Geometry check sheet. Reference: the model listing, model coordinates, mm. Face numbers are marked on the shaded views. A direction names the side the tool comes from. Coordinates: 2 decimals unless noted, no trailing zeros. Loops run counter-clockwise (first coordinate to the right, second up) from the corner with the lowest first, then second, coordinate; pieces in that order, holes last. Notation, with made-up numbers: (-4.5, -1.75) -> (38.5, -1.75) arc R36 cw to (38.5, 35.25) -> close; hole circle Ø3 at (85.5, 68.25). An arc over 180 degrees is marked (long way). Answer as a JSON object with one key per item and string values.
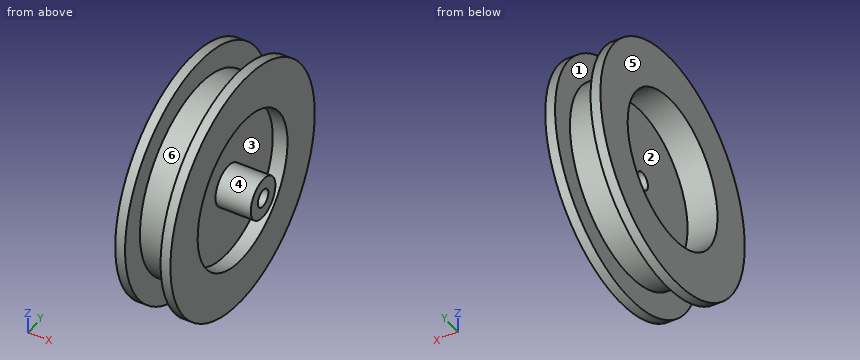
from build123d import *

# Parameters (mm, degrees)
SKETCH1_R           = 76.2635
BOSS_EXTRUDE1_DEPTH = 17.3228
SKETCH2_R           = 47.46625
CUT_EXTRUDE1_DEPTH  = 9.271
CUT_EXTRUDE2_START  = -15.8496
SKETCH2_2_R         = 47.46625
CUT_EXTRUDE2_DEPTH  = 18.796
CUT_EXTRUDE3_START  = -6.1722
SKETCH3_OUTSIDE_W   = 198.222
SKETCH3_OUTSIDE_H   = 198.222
SKETCH3_OUTSIDE_R   = 60.5536
CUT_EXTRUDE3_DEPTH  = 22.3012
SKETCH4_R           = 13.0175
BOSS_EXTRUDE2_DEPTH = 22.1615
SKETCH5_R           = 5.59435
CUT_EXTRUDE4_DEPTH  = 118.864004971


with BuildPart() as part:
    # Sketch1 → Boss-Extrude1 (new, symmetric)
    with BuildSketch(Plane(origin=(0, 0, 0), x_dir=(0, 0, -1), z_dir=(1, 0, 0))):
        Circle(SKETCH1_R)
    extrude(amount=BOSS_EXTRUDE1_DEPTH, both=True)

    # Sketch2 → Cut-Extrude1 (cut)
    with BuildSketch(Plane(origin=(17.3228, 0, 0), x_dir=(0, 0, -1), z_dir=(1, 0, 0))):
        Circle(SKETCH2_R)
    extrude(amount=-CUT_EXTRUDE1_DEPTH, mode=Mode.SUBTRACT)

    # Sketch2<2> → Cut-Extrude2 (cut)
    with BuildSketch(Plane(origin=(17.3228, 0, 0), x_dir=(0, 0, -1), z_dir=(1, 0, 0)).offset(CUT_EXTRUDE2_START)):
        Circle(SKETCH2_2_R)
    extrude(amount=-CUT_EXTRUDE2_DEPTH, mode=Mode.SUBTRACT)

    # Sketch3 outside → Cut-Extrude3 (cut)
    with BuildSketch(Plane(origin=(17.3228, 0, 0), x_dir=(0, 0, -1), z_dir=(1, 0, 0)).offset(CUT_EXTRUDE3_START)):
        Rectangle(SKETCH3_OUTSIDE_W, SKETCH3_OUTSIDE_H)
        Circle(SKETCH3_OUTSIDE_R, mode=Mode.SUBTRACT)
    extrude(amount=-CUT_EXTRUDE3_DEPTH, mode=Mode.SUBTRACT)

    # Sketch4 → Boss-Extrude2 (add)
    with BuildSketch(Plane(origin=(8.0518, 0, 0), x_dir=(0, 0, -1), z_dir=(1, 0, 0))):
        Circle(SKETCH4_R)
    extrude(amount=BOSS_EXTRUDE2_DEPTH)

    # Sketch5 → Cut-Extrude4 (cut, through all)
    with BuildSketch(Plane(origin=(30.2133, 0, 0), x_dir=(0, 0, -1), z_dir=(1, 0, 0))):
        Circle(SKETCH5_R)
    extrude(amount=-CUT_EXTRUDE4_DEPTH, mode=Mode.SUBTRACT)


solid = part.part
1. Depth check by flat-ended pin: P1, Ø1.5, axis at x = 10.5, y = 8.5, coming from the -Z side; P2, Ø4, axis at x = -7.5, z = -28, coming from the -Y side; P3, Ø2, axis at x = 14.5, y = -6.5, coming from the -Z side; P4, Ø9, axis at y = 0, z = 0, coming from the +X side. Enter the tip coordinate at first touch or a pass-through.
Evaluation:
{"P1": "stops at z = -75.83", "P2": "stops at y = -54.69", "P3": "stops at z = -76.06", "P4": "passes through"}
2. Tool access check on the marked faces 1, 2 and 3. Record the directions out of +Z, -Z, +X, -X, +Y, -Y that give a thin tool (end or side, any length) a straight path to the whole face; none if there is none.
Evaluation:
{"face 1": "none", "face 2": "-X", "face 3": "+X"}
3. Mould release check, pull along Y, two halves, no side actions. Record for the marked faces 4, 5 and 6: released by +Y, released by -Y, zero draft, split by the parting line, or undercut.
Evaluation:
{"face 4": "undercut", "face 5": "zero draft", "face 6": "split by the parting line"}
4. Section check D-D, the plane z = -53. Record the boundary of the cut face in (x, y).
Evaluation:
{"outline": "(-17.32, -54.84) -> (-11.15, -54.84) -> (-11.15, -29.29) -> (11.15, -29.29) -> (11.15, -54.84) -> (17.32, -54.84) -> (17.32, 54.84) -> (11.15, 54.84) -> (11.15, 29.29) -> (-11.15, 29.29) -> (-11.15, 54.84) -> (-17.32, 54.84) -> close"}
5. Thickness scan on probe 1 along Y at (x, z) = (-8.75, 0); probe 2 along Y at (x, z) = (21.75, 0); probe 3 along X at (y, z) = (-46.5, -39). Record the ranges inside material, lowest first. Write a range as from..to.
Evaluation:
{"probe 1": "y = -60.55..-47.47, 47.47..60.55", "probe 2": "y = -13.02..-5.59, 5.59..13.02", "probe 3": "x = -17.32..-11.15, 11.15..17.32"}
6. Section check C-C, the plane x = 24.5. Record the boundary of the cut face in (y, z) (1 decimal), then the cut area to 3 significant figures.
Evaluation:
{"outline": "circle Ø26 at (0, 0); hole circle Ø11.2 at (0, 0)", "area": "434 mm^2"}
7. Section check A-A, the plane z = 0. Record the boundary of the cut face in (x, y), then the cut area to 3 significant figures.
Evaluation:
{"outline": "(-17.32, -76.26) -> (-11.15, -76.26) -> (-11.15, -60.55) -> (11.15, -60.55) -> (11.15, -76.26) -> (17.32, -76.26) -> (17.32, -47.47) -> (8.05, -47.47) -> (8.05, -13.02) -> (30.21, -13.02) -> (30.21, -5.59) -> (1.47, -5.59) -> (1.47, -47.47) -> (-17.32, -47.47) -> close; (-17.32, 47.47) -> (1.47, 47.47) -> (1.47, 5.59) -> (30.21, 5.59) -> (30.21, 13.02) -> (8.05, 13.02) -> (8.05, 47.47) -> (17.32, 47.47) -> (17.32, 76.26) -> (11.15, 76.26) -> (11.15, 60.55) -> (-11.15, 60.55) -> (-11.15, 76.26) -> (-17.32, 76.26) -> close", "area": "2,170 mm^2"}
